Read the model definition and answer for the solid it produces. Units are mm, in the model's axes. A direction names the side the tool comes from. Coordinates: 2 decimals unless noted, no trailing zeros. Write each loop counter-clockwise with the first axis right and the second up, starting at its lowest first coordinate (ties: lowest second). Pieces come first, ordered by that corner, then holes.
(1) Straight lines are drawn through the part: line 1 along Y through (x, z) = (3.75, 21); line 2 along X through (y, z) = (-5.5, 9.5); line 3 along Y through (x, z) = (3.25, 51). For each, find the intervals that lie inside material, in ascending order.
(2) Determine the mould class of faces 1 (the flat face through (-6, -5, 37)), 2 (the flat face through (-10, -7, 37)), 3 (the flat face through (8, 5, 37)), 4 (the flat face through (7, -10, 37)) for opening direction X: pulls with the +X half, pulls with the -X half, needs draft (parallel to the pull), parting line crosses it, or undercut.
(3) The part is cut by section A-A, the plane y = 1.75. Determine the outline of the cut face in (x, z).
(4) Given pin 1 (3 mm diameter, centred on x = -0.5, z = 22, fed in from +Y); pin 2 (1 mm diameter, centred on x = -3, z = 54.5, fed in from -Y); pin 3 (6.5 mm diameter, centred on y = -0.5, z = 35, fed in from +X), each flat-ended and moving along its own axis, determine where each tip first touches the part or whether it passes through.
(5) Which of the six approach directions +Z, -Z, +X, -X, +Y, -Y give full straight-line access (tool end or side, diameter ignored) to faces 5 (the flat face through (6, -5, 37)), 6 (the flat face through (-9, -4, 37)), 7 (the flat face through (9, 4, 37)), 8 (the flat face through (4, 9, 37))?
```python
from build123d import *

# Parameters (mm, degrees)
F1_DEPTH = 50
F2_DEPTH = 25


with BuildPart() as f1:
    # F0 (on Top) → F1 (new body)
    with BuildSketch(Plane.XY):
        Polygon((4, 3), (4, 4), (3, 4), (-3, 4), (-4, 4), (-4, 3), (-4, -3), (-4, -4), (-3, -4), (3, -4), (4, -4), (4, -3), align=None)
        Polygon((-8, -3), (-10, -5), (-10, -10), (-4, -4), (-4, -3), (-8, -7), align=None)
        Polygon((-10, -10), (-5, -10), (-3, -8), (-7, -8), (-3, -4), (-4, -4), align=None)
        Polygon((5, -10), (10, -10), (4, -4), (3, -4), (7, -8), (3, -8), align=None)
        Polygon((10, -10), (10, -5), (8, -3), (8, -7), (4, -3), (4, -4), align=None)
        Polygon((10, 5), (10, 10), (4, 4), (4, 3), (8, 7), (8, 3), align=None)
        Polygon((4, 4), (10, 10), (5, 10), (3, 8), (7, 8), (3, 4), align=None)
        Polygon((-3, 8), (-5, 10), (-10, 10), (-4, 4), (-3, 4), (-7, 8), align=None)
        Polygon((-4, 4), (-10, 10), (-10, 5), (-8, 3), (-8, 7), (-4, 3), align=None)
    extrude(amount=F1_DEPTH)

    # F2 (add): a face of the model
    f2_faces = [f1.faces().sort_by_distance(p)[0] for p in [
        (0, 0, 50),
    ]]
    extrude(f2_faces, amount=F2_DEPTH)


solid = f1.part
```
Computed:
1. line 1: y = -8.75 to -8, -4.75 to 4.75, 8 to 8.75
1. line 2: x = -10 to -8, -6.5 to -4.5, 4.5 to 6.5, 8 to 10
1. line 3: y = -8.25 to -8, -4.25 to 4.25, 8 to 8.25
2. face 1: undercut
2. face 2: pulls with the -X half
2. face 3: undercut
2. face 4: needs draft
3. outline: (-4, 0) - (4, 0) - (4, 75) - (-4, 75) - close
4. pin 1: stops at y = 4
4. pin 2: stops at y = -8.5
4. pin 3: stops at x = 8.75
5. face 5: +Z, -Z
5. face 6: +Z, -Z, -X
5. face 7: +Z, -Z, +X
5. face 8: +Z, -Z, +Y
